from build123d import *

# Parameters (mm, degrees)
SKETCH1_R            = 35.03125
SKETCH1_R_2          = 30.03125
BOSS_EXTRUDE1_DEPTH  = 30
M3_CLEARANCE_HOLE2_D = 3.4
M3_CLEARANCE_HOLE3_D = 3.4
BOSS_EXTRUDE2_DEPTH  = 5
M3_CLEARANCE_HOLE4_D = 3.4
SKETCH14_W           = 15
SKETCH14_H           = 123.928098147
CUT_EXTRUDE1_DEPTH   = 15


with BuildPart() as part:
    # Sketch1 → Boss-Extrude1 (new body)
    with BuildSketch(Plane(origin=(0, 0, 0), x_dir=(0, 0, -1), z_dir=(1, 0, 0))):
        Circle(SKETCH1_R)
        Circle(SKETCH1_R_2, mode=Mode.SUBTRACT)
    extrude(amount=BOSS_EXTRUDE1_DEPTH)

    # M3 Clearance Hole2 (through all)
    with Locations(Plane(origin=(0, 35.03125, 0), x_dir=(1, 0, 0), z_dir=(0, 1, 0))):
        with Locations((5, 0)):
            Hole(M3_CLEARANCE_HOLE2_D / 2)

    # M3 Clearance Hole3 (through all)
    with Locations(Plane.XY.offset(35.03125)):
        with Locations((5, 0)):
            Hole(M3_CLEARANCE_HOLE3_D / 2)

    # Sketch9 → Boss-Extrude2 (add)
    with BuildSketch(Plane(origin=(30, 0, 0), x_dir=(0, 0, -1), z_dir=(1, 0, 0))):
        with BuildLine():
            Line((14, 71.5), (45, 71.5))
            Line((45, 71.5), (45, -71.5))
            Line((45, -71.5), (14, -71.5))
            Line((14, -71.5), (14, -26.568326567))
            ThreePointArc((14, -26.568326567), (30.03125, 0), (14, 26.568326567))
            Line((14, 26.568326567), (14, 71.5))
        make_face()
    extrude(amount=BOSS_EXTRUDE2_DEPTH)

    # M3 Clearance Hole4 (through all)
    with Locations(Plane(origin=(35, 0, 0), x_dir=(0, 0, -1), z_dir=(1, 0, 0))):
        with Locations((24, 30.034163283), (24, 65.5), (24, -65.5), (24, -30.034163283)):
            Hole(M3_CLEARANCE_HOLE4_D / 2)

    # Sketch14 → Cut-Extrude1 (cut)
    with BuildSketch(Plane(origin=(30, 0, 0), x_dir=(0, 0, -1), z_dir=(1, 0, 0))):
        with Locations((0, 15.044796635)):
            Rectangle(SKETCH14_W, SKETCH14_H)
    extrude(amount=-CUT_EXTRUDE1_DEPTH, mode=Mode.SUBTRACT)


solid = part.part
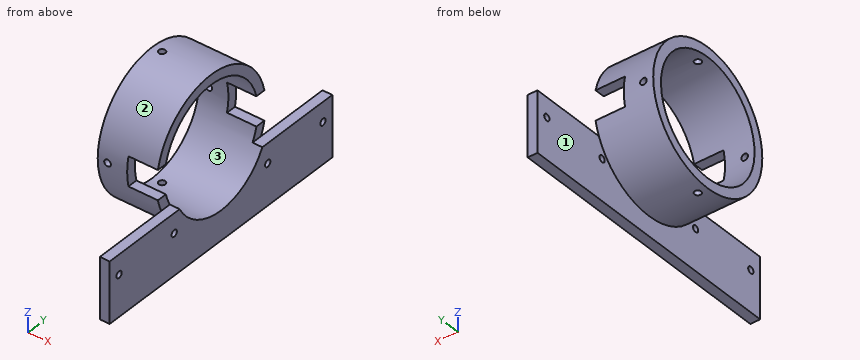
Build history of the part. All positions in model axes, mm. Face numbers are marked on the shaded views. Coordinates: 2 decimals unless noted, no trailing zeros. Write each loop counter-clockwise with the first axis right and the second up, starting at its lowest first coordinate (ties: lowest second). Pieces come first, ordered by that corner, then holes.
(1) Mould opens along Y. For the marked faces 1, 2 and 3 say: pulls with the +Y half, pulls with the -Y half, needs draft (parallel to the pull), parting line crosses it, or undercut.
(2) Drill centre lines: line 1 (Y direction, x = 31.9, z = -24); line 2 (X direction, y = 0, z = -33.4); line 3 (Z direction, x = 20.5, y = 1). Where is each one in solid material? Low to high.
(3) Cut at C-C on x = 28. List the corners of the cut face in (y, z).
(4) Cut at B-B on y = 65.5. List the corners of the cut face in (x, z).
(5) Cut at A-A on z = 0. List the corners of the cut face in (x, y).
(6) Cut at D-D on y = 0. List the corners of the cut face in (x, z).
(7) Pin check, flat tips, straight feed: pin 1 Ø4 at (x, z) = (5, -33.5) entering from +Y; pin 2 Ø5 at (x, y) = (23.5, -1) entering from -Z; pin 3 Ø5 at (x, z) = (5, -34.5) entering from +Y; pin 4 Ø2 at (x, z) = (5, 0) entering from -Y. Stop position of each tip, or through.
Working result:
1. face 1: needs draft
1. face 2: parting line crosses it
1. face 3: undercut
2. line 1: y = -71.5 to -67.2, -63.8 to -31.73, -28.33 to -18.05, 18.05 to 28.33, 31.73 to 63.8, 67.2 to 71.5
2. line 2: x = 0 to 3.3, 6.7 to 35
2. line 3: z = -35.02 to -30.01, 30.01 to 35.02
3. outline: (-34.22, -7.5) arc R35.03 ccw to (34.22, -7.5) - (29.08, -7.5) arc R30.03 cw to (-29.08, -7.5) - close; (-34.22, 7.5) - (-29.08, 7.5) arc R30.03 cw to (29.08, 7.5) - (34.22, 7.5) arc R35.03 ccw to start
4. outline: (30, -45) - (35, -45) - (35, -25.7) - (30, -25.7) - close; (30, -22.3) - (35, -22.3) - (35, -14) - (30, -14) - close
5. outline: (0, -35.03) - (3.3, -35.03) - (3.3, -30.03) - (0, -30.03) - close; (0, 30.03) - (3.3, 30.03) - (3.3, 35.03) - (0, 35.03) - close; (6.7, -35.03) - (15, -35.03) - (15, -30.03) - (6.7, -30.03) - close; (6.7, 30.03) - (15, 30.03) - (15, 35.03) - (6.7, 35.03) - close
6. outline: (0, -35.03) - (3.3, -35.03) - (3.3, -30.03) - (0, -30.03) - close; (0, 30.03) - (3.3, 30.03) - (3.3, 35.03) - (0, 35.03) - close; (6.7, -35.03) - (30, -35.03) - (30, -45) - (35, -45) - (35, -30.03) - (6.7, -30.03) - close; (6.7, 30.03) - (30, 30.03) - (30, 35.03) - (6.7, 35.03) - close
7. pin 1: stops at y = 15.33
7. pin 2: stops at z = -35.03
7. pin 3: stops at y = 14.25
7. pin 4: passes through
